The model under review builds one solid part; all positions refer to its coordinate system, in mm. Face numbers are marked on the shaded views. Give positions to 0.01 mm unless a question says otherwise; leave off trailing zeros. Order: outer loops, then holes, each group sorted by start corner. A loop starts at its lowest first (then second) coordinate and runs counter-clockwise, first axis right, second up. Notation, with made-up numbers: (-15.75, -35) - (-9.75, -35) arc R16 cw to (-9.75, -29) - close; hole circle Ø2 at (1, -39.5). An arc over 180 degrees is marked (long way). Put each result on its own line as item: value.
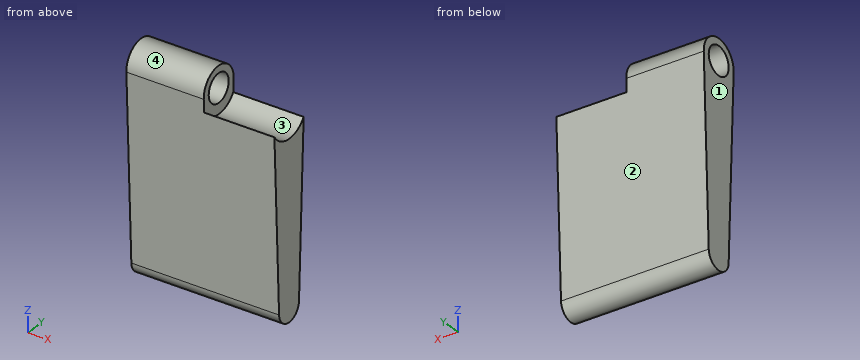
```python
from build123d import *

# Parameters (mm, degrees)
BOSS_EXTRUDE1_DEPTH = 16.46682
SKETCH2_R           = 2.7432
CUT_EXTRUDE1_DEPTH  = 7.84098
SKETCH3_R           = 1.56718
CUT_EXTRUDE2_DEPTH  = 9.62584


with BuildPart() as part:
    # Sketch1 → Boss-Extrude1 (new body)
    with BuildSketch(Plane(origin=(0, 0, 0), x_dir=(0, 0, -1), z_dir=(1, 0, 0))):
        with BuildLine():
            Line((-10.13615668, 2.350298814), (10.23492888, 1.566019836))
            ThreePointArc((10.23492888, 1.566019836), (11.741817718, 0), (10.23492888, -1.566019836))
            Line((10.23492888, -1.566019836), (-10.13615668, -2.350298814))
            ThreePointArc((-10.13615668, -2.350298814), (-12.578682282, 0), (-10.13615668, 2.350298814))
        make_face()
    extrude(amount=-BOSS_EXTRUDE1_DEPTH)

    # Sketch2 → Cut-Extrude1 (cut)
    with BuildSketch(Plane(origin=(0, 0, 0), x_dir=(0, 0, -1), z_dir=(1, 0, 0))):
        with Locations((-10.226642282, 0)):
            Circle(SKETCH2_R)
    extrude(amount=-CUT_EXTRUDE1_DEPTH, mode=Mode.SUBTRACT)

    # Sketch3 → Cut-Extrude2 (cut, through all)
    with BuildSketch(Plane(origin=(-7.84098, 0, 0), x_dir=(0, 0, -1), z_dir=(1, 0, 0))):
        with Locations((-10.226642282, 0)):
            Circle(SKETCH3_R)
    extrude(amount=-CUT_EXTRUDE2_DEPTH, mode=Mode.SUBTRACT)


solid = part.part
```
(1) Wall thickness on L1, parallel to Z at x = -12.5, y = -0.1; L2, parallel to Y at x = -8.25, z = -10.25; L3, parallel to X at y = 2.05, z = 10.5: over which ranges is each line inside the solid? List them lowest first.
The answers:
L1: -11.74 to 8.66, 11.79 to 12.58
L2: -1.57 to 1.57
L3: -16.47 to -7.84
(2) The part is to be moulded in two halves that separate along Y. For the marked faces 1, 2, 3 and 4, say which applies: pulls with the +Y half, pulls with the -Y half, needs draft (parallel to the pull), parting line crosses it, or undercut.
The answers:
face 1: needs draft
face 2: pulls with the +Y half
face 3: undercut
face 4: parting line crosses it
(3) Clearance check with flat-ended pins moving along their axes: pin 1 Ø2 at (x, y) = (-4.5, -0.5) entering from +Z; pin 2 Ø6 at (x, z) = (-11, -6.5) entering from -Y; pin 3 Ø1 at (x, y) = (-3, -1) entering from -Z. State where each tip first meets the part, or that it passes through.
The answers:
pin 1: z = 7.93
pin 2: y = -1.83
pin 3: z = -11.66
(4) Take a section at C-C, the plane z = 11. Write out the cut boundary in (x, y), then the cut area to 3 significant figures.
The answers:
outline: (-16.47, -2.22) - (-7.84, -2.22) - (-7.84, -1.36) - (-16.47, -1.36) - close; (-16.47, 1.36) - (-7.84, 1.36) - (-7.84, 2.22) - (-16.47, 2.22) - close
area: 14.8 mm^2
(5) Take a section at A-A, the plane y = 0. Write out the cut boundary in (x, z), then the cut area to 3 significant figures.
The answers:
outline: (-16.47, -11.74) - (0, -11.74) - (0, 7.48) - (-7.84, 7.48) - (-7.84, 8.66) - (-16.47, 8.66) - close; (-16.47, 11.79) - (-7.84, 11.79) - (-7.84, 12.58) - (-16.47, 12.58) - close
area: 333 mm^2
(6) Take a section at D-D, the plane x = -5.5. Write out the cut boundary in (y, z).
The answers:
outline: (-2.3, 8.73) - (-1.57, -10.23) arc R1.57 ccw to (1.57, -10.23) - (2.3, 8.73) arc R2.74 cw to start
(7) Take a section at B-B, the plane x = -12.75. Write out the cut boundary in (y, z).
The answers:
outline: (-2.35, 10.14) - (-1.57, -10.23) arc R1.57 ccw to (1.57, -10.23) - (2.35, 10.14) arc R2.35 ccw (long way) to start; hole circle Ø3.13 at (0, 10.23)
